The model under review builds one solid part; all positions refer to its coordinate system, in mm. Face numbers are marked on the shaded views. A direction names the side the tool comes from. Round coordinates to 2 decimals unless told otherwise and drop trailing zeros. Order: outer loops, then holes, each group sorted by start corner. A loop starts at its lowest first (then second) coordinate and runs counter-clockwise, first axis right, second up.
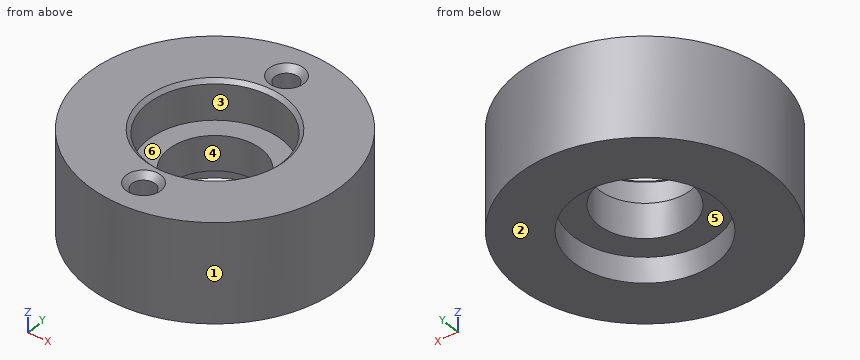
Autodesk Inventor part; units mm, degrees
ref_plane "YZ Plane" through (0, 0, 0) normal (1, 0, 0) x (0, 1, 0)
ref_plane "XZ Plane" through (0, 0, 0) normal (0, 1, 0) x (-1, 0, 0)
ref_plane "XY Plane" through (0, 0, 0) normal (0, 0, 1) x (1, 0, 0)
sketch "Эскиз1" plane through (0, 0, 0) normal (0, 0, 1) x (1, 0, 0)
  circle A0 centre (0, 0) radius 55
  circle A1 centre (0, 0) radius 20
  dimension "d0" = 110
  dimension "d1" = 40
extrude "Выдавливание1" add sketch "Эскиз1" along normal blind 43
sketch "Эскиз2" plane through (0, 0, 43) normal (0, 0, 1) x (1, 0, 0)
  circle A0 centre (0, 0) radius 55
  circle A1 centre (0, 0) radius 29
  dimension "d6" = 58
extrude "Выдавливание2" cut sketch "Эскиз2" against normal blind 17 contours A1
sketch "Эскиз3" plane through (0, 0, 0) normal (0, 0, -1) x (-1, 0, 0)
  circle A0 centre (0, 0) radius 31
  dimension "d9" = 62
extrude "Выдавливание3" cut sketch "Эскиз3" against normal blind 11
sketch "Эскиз4" plane through (0, 0, 43) normal (0, 0, 1) x (1, 0, 0)
  circle A0 centre (0, 0) radius 40
  line L0 (0, 0) -> (0, 40)
  circle A1 centre (0, 0) radius 55
  dimension "d12" = 80
hole "Отверстие1" at (0, 40, 43) direction (0, 0, -1) diameter 10.106 depth 38.3 tip angle 118
pattern_circular "Круговой массив1" count 2 over 360 about axis through (0, 0, 11) along (0, 0, -1) of "Отверстие1"
chamfer "Фаска2" distance 1.6 angle 45 1 edges at (-29, 0, 43)
chamfer "Фаска3" distance 2.5 angle 45 2 edges at (0, 45.053, 43) (0, -45.053, 43)
sketch "Эскиз5" plane through (0, 0, 43) normal (0, 0, 1) x (1, 0, 0)
  point P0 (0, 40)
  point P1 (-62.4077, 41.077)
properties part number "Корпус"
(1) We need section C-C (x = -36.5). Give the boundary of the cut face in (y, z), and give its area (3 significant figures).
(2) Tool access review of the marked faces 4, 5 and 6: name each direction out of +Z, -Z, +X, -X, +Y, -Y from which nothing blocks a thin tool from reaching the whole face with its end or side.
(3) To check wall thickness, follow L1, parallel to Y at x = 0, z = 2.5; L2, parallel to X at y = 3.5, z = 6; L3, parallel to Y at x = 8, z = 20. State the ranges of each line that lie inside material, in increasing order.
(4) We need section B-B (z = 33.5). Give the boundary of the cut face in (x, y), and give its area (3 significant figures).
(5) We need section A-A (y = 0). Give the boundary of the cut face in (x, z), and give its area (3 significant figures).
(6) We need section D-D (z = 12.5). Give the boundary of the cut face in (x, y).
(7) Clearance check with flat-ended pins moving along their axes: P1, Ø9, axis at x = 0, y = -40, coming from the +Z side; P2, Ø8, axis at x = 3, z = 36.5, coming from the -Y side; P3, Ø17.5, axis at x = 5.5, y = -6.5, coming from the +Z side; P4, Ø12, axis at y = 28.5, z = 7.5, coming from the -X side. State where each tip first meets the part, or that it passes through.
(8) The part is to be moulded in two halves that separate along X. For the marked faces 1, 2 and 3, say which applies: pulls with the +X half, pulls with the -X half, needs draft (parallel to the pull), parting line crosses it, or undercut.
Verdict:
1. outline: (-41.14, 0) - (41.14, 0) - (41.14, 43) - (-41.14, 43) - close
1. area: 3,540 mm2
2. face 4: +Z, -Z
2. face 5: -Z
2. face 6: +Z
3. L1: y = -55 to -41.39, -38.61 to -31, 31 to 38.61, 41.39 to 55
3. L2: x = -54.89 to -30.8, 30.8 to 54.89
3. L3: y = -54.42 to -18.33, 18.33 to 54.42
4. outline: circle Ø110 at (0, 0); hole circle Ø58 at (0, 0); hole circle Ø10.11 at (0, -40); hole circle Ø10.11 at (0, 40)
4. area: 6,700 mm2
5. outline: (-55, 0) - (-31, 0) - (-31, 11) - (-20, 11) - (-20, 26) - (-29, 26) - (-29, 41.4) - (-30.6, 43) - (-55, 43) - close; (20, 11) - (31, 11) - (31, 0) - (55, 0) - (55, 43) - (30.6, 43) - (29, 41.4) - (29, 26) - (20, 26) - close
5. area: 2,460 mm2
6. outline: circle Ø110 at (0, 0); hole circle Ø40 at (0, 0); hole circle Ø10.11 at (0, -40); hole circle Ø10.11 at (0, 40)
7. P1: stops at z = 4.37
7. P2: stops at y = -55
7. P3: passes through
7. P4: stops at x = -50.19
8. face 1: parting line crosses it
8. face 2: needs draft
8. face 3: undercut
